Could you check a few things on this drawing? It's one solid part, dimensions in mm from its lowest x, y, z. A direction names the side the tool comes from. Give positions to 0.01 mm unless a question says otherwise; leave off trailing zeros. Order: outer loops, then holes, each group sorted by start corner. A loop starts at its lowest first (then second) coordinate and runs counter-clockwise, first axis right, second up.
(1) On a 3-axis mill with a long thin cutter (end or side, diameter ignored), from which of +Z, -Z, +X, -X, +Y, -Y can I reach the whole of each face in a straight line? I mean the marked faces 1, 2, 3 and 4. Say none if no direction works.
(2) Imagine slicing it at D-D, the plane y = 2.2. Write out the boundary of the cut face in (x, z).
(3) Imagine slicing it at C-C, the plane x = 5.75. Write out the boundary of the cut face in (y, z) (3 decimals), then the cut area to 3 significant figures.
(4) Imagine slicing it at B-B, the plane z = 3.1. Write out the boundary of the cut face in (x, y), then the cut area to 3 significant figures.
(5) If I drill on probe 1 along X at (y, z) = (2.3, 1.3); probe 2 along Y at (x, z) = (1.5, 2.65); probe 3 along Y at (x, z) = (6.5, 4.5), over which ranges is the centre line in solid material (lowest first)?
(6) Imagine slicing it at A-A, the plane y = 4.3. Write out the boundary of the cut face in (x, z), then the cut area to 3 significant figures.
(7) Will these pins go through, and if not, where does the flat tip stop? pin 1 (1 mm diameter, centred on x = 1, z = 4, fed in from +Y); pin 2 (0.8 mm diameter, centred on y = 2.5, z = 1, fed in from -X); pin 3 (2 mm diameter, centred on x = 3, z = 3, fed in from -Y); pin 4 (1.5 mm diameter, centred on y = 4.5, z = 3, fed in from -X).
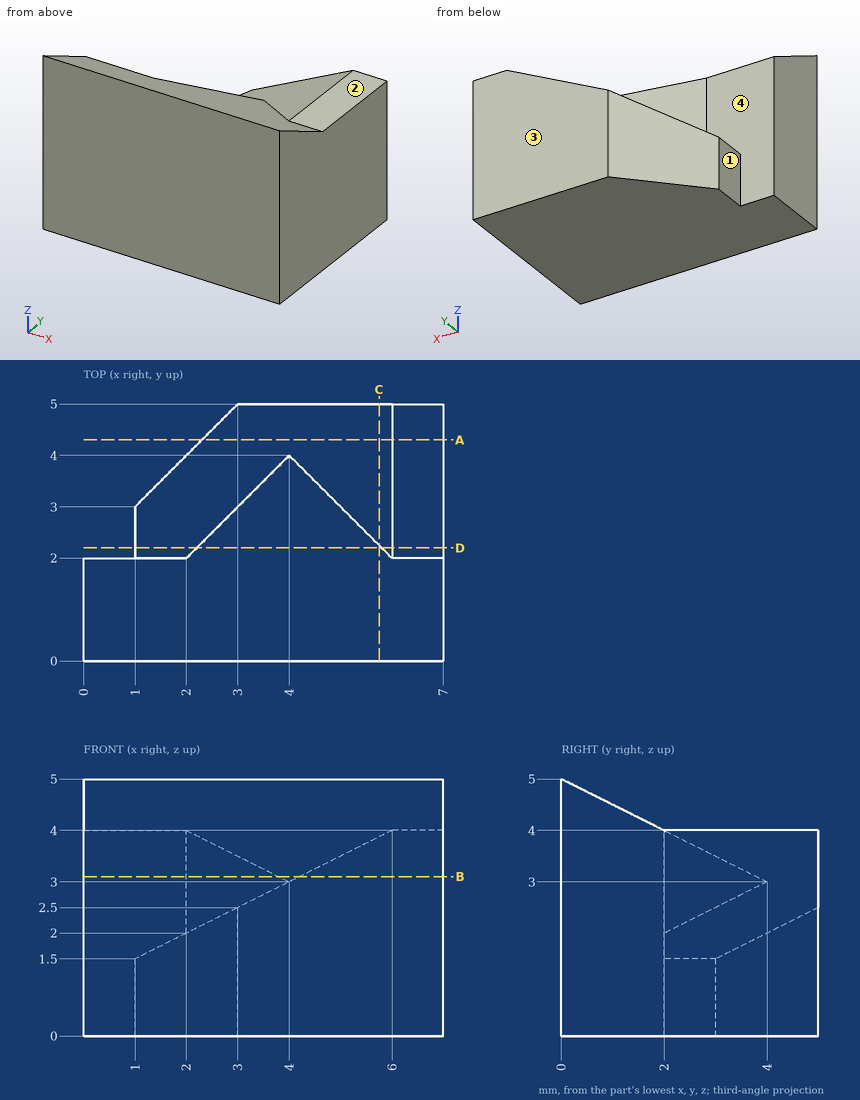
Answer block:
1. face 1: +Z, -Z, -X, +Y
1. face 2: +Z, +X, -X, +Y
1. face 3: +Z, -Z, +X, -X, +Y
1. face 4: +Z, -X, +Y
2. outline: (1, 0) - (7, 0) - (7, 4) - (6, 4) - (5.8, 3.9) - (2.2, 3.9) - (2.2, 2.1) - (1, 1.5) - close
3. outline: (0, 0) - (5, 0) - (5, 3.875) - (2.25, 3.875) - (0, 5) - close
3. area: 20.6 mm2
4. outline: (0, 0) - (7, 0) - (7, 5) - (4.2, 5) - (4.2, 3.8) - (3.8, 3.8) - (2, 2) - (0, 2) - close
4. area: 24.7 mm2
5. probe 1: x = 1 to 7
5. probe 2: y = 0 to 2
5. probe 3: y = 0 to 1
6. outline: (2.3, 0) - (7, 0) - (7, 4) - (6, 4) - (2.3, 2.15) - close
6. area: 15.4 mm2
7. pin 1: stops at y = 2
7. pin 2: stops at x = 1
7. pin 3: stops at y = 0
7. pin 4: stops at x = 2.5
